```python
from build123d import *

# Parameters (mm, degrees)
SKETCH021_W             = 85.5
SKETCH021_H             = 85.5
SKETCH021_W_2           = 73.5
SKETCH021_H_2           = 73.5
PAD009006_DEPTH         = 11
SKETCH022_W             = 85.5
SKETCH022_H             = 85.5
SKETCH022_R             = 25.5
PAD009007_DEPTH         = 2
SKETCH023_R             = 1.5
POCKET003002_DEPTH      = 13.001
SKETCH024_R             = 1.5
POCKET003003_DEPTH      = 5
FILLET003_R             = 3
SKETCH025_W             = 45.5
SKETCH025_H             = 5
POCKET003004_DEPTH      = 85.501
POCKET003004_DEPTH_BACK = 0.001
SKETCH026_W             = 45.5
SKETCH026_H             = 5
POCKET003005_DEPTH      = 85.501


with BuildPart() as part:
    # Sketch021 → Pad009006 (new body)
    with BuildSketch(Plane.XY):
        Rectangle(SKETCH021_W, SKETCH021_H)
        Rectangle(SKETCH021_W_2, SKETCH021_H_2, mode=Mode.SUBTRACT)
    extrude(amount=PAD009006_DEPTH)

    # Sketch022 (on Face10 of Pad009006) → Pad009007 (join)
    with BuildSketch(Plane.XY.offset(11)):
        Rectangle(SKETCH022_W, SKETCH022_H)
        Circle(SKETCH022_R, mode=Mode.SUBTRACT)
    extrude(amount=PAD009007_DEPTH)

    # Sketch023 (on Face4 of Pad009007) → Pocket003002 (cut, through all)
    with BuildSketch(Plane(origin=(0, 0, 0), x_dir=(1, 0, 0), z_dir=(0, 0, -1))):
        with Locations((-39.235281, 39.235281)):
            Circle(SKETCH023_R)
        with Locations((39.235281, 39.235281)):
            Circle(SKETCH023_R)
        with Locations((39.235281, -39.235281)):
            Circle(SKETCH023_R)
        with Locations((-39.235281, -39.235281)):
            Circle(SKETCH023_R)
    extrude(amount=-POCKET003002_DEPTH, mode=Mode.SUBTRACT)

    # Sketch024 (on Face17 of Pocket003002) → Pocket003003 (cut)
    with BuildSketch(Plane.XY.offset(13)):
        with Locations((-30, 30)):
            Circle(SKETCH024_R)
        with Locations((30, 30)):
            Circle(SKETCH024_R)
        with Locations((30, -30)):
            Circle(SKETCH024_R)
        with Locations((-30, -30)):
            Circle(SKETCH024_R)
    extrude(amount=-POCKET003003_DEPTH, mode=Mode.SUBTRACT)

    # Fillet003
    fillet003_edges = [part.edges().sort_by_distance(p)[0] for p in [
        (42.75, 42.75, 5.5),
        (-42.75, 42.75, 5.5),
        (-42.75, -42.75, 5.5),
        (42.75, -42.75, 5.5),
    ]]
    fillet(fillet003_edges, radius=FILLET003_R)

    # Sketch025 (on Face1 of Fillet003) → Pocket003004 (cut, two sides)
    with BuildSketch(Plane(origin=(0, 42.75, 0), x_dir=(-1, 0, 0), z_dir=(0, 1, 0))) as pocket003004_sk:
        with Locations((0, 2.5)):
            Rectangle(SKETCH025_W, SKETCH025_H)
    extrude(amount=-POCKET003004_DEPTH, mode=Mode.SUBTRACT)
    extrude(pocket003004_sk.sketch, amount=POCKET003004_DEPTH_BACK, mode=Mode.SUBTRACT)

    # Sketch026 (on Face19 of Pocket003004) → Pocket003005 (cut, through all)
    with BuildSketch(Plane.YZ.offset(42.75)):
        with Locations((0, 2.5)):
            Rectangle(SKETCH026_W, SKETCH026_H)
    extrude(amount=-POCKET003005_DEPTH, mode=Mode.SUBTRACT)


solid = part.part
```
Geometry check sheet. Reference: the model listing, model coordinates, mm. A direction names the side the tool comes from. Give positions to 0.01 mm unless a question says otherwise; leave off trailing zeros. Write each loop counter-clockwise with the first axis right and the second up, starting at its lowest first coordinate (ties: lowest second). Pieces come first, ordered by that corner, then holes.
1) Section check A-A, the plane y = -30. Record the boundary of the cut face in (x, z).
2) Access from +Z, -Z, +X, -X, +Y, -Y to the whole of each face (thin tool, end or side, straight path). Record for faces 5 (the flat face through (0, 40, 5)), 6 (the flat face through (-36.75, -1, 7)), 7 (the flat face through (40, 22.75, 2)).
3) Gauge pin test, flat ends, axial feed: pin 1 (3.5 mm diameter, centred on x = 30, y = 30, fed in from -Z); pin 2 (5 mm diameter, centred on x = -38.5, y = -10, fed in from -Z); pin 3 (1.8 mm diameter, centred on x = -39.24, y = -39.24, fed in from +Z); pin 4 (1.5 mm diameter, centred on y = -41, z = 2, fed in from +X). Record the tip position at first contact, or that the pin passes through.
4) Material ranges on L1, parallel to Y at x = -30, z = 12; L2, parallel to Y at x = 0, z = 12.6; L3, parallel to X at y = -27.5, z = 8.5, recorded low to high.
5) Section check C-C, the plane y = 0. Record the boundary of the cut face in (x, z), and give its area (3 significant figures).
6) Release check for a two-part mould opening along Y. For faces 1 (the cylindrical face through (-41.89, -41.85, 6.59)), 2 (the flat face through (-1, -36.75, 7)), 3 (the flat face through (-22.75, 40, 2)), 4 (the flat face through (-1, 42.75, 8)) record: pulls with the +Y half, pulls with the -Y half, needs draft (parallel to the pull), parting line crosses it, or undercut.
Computed:
1. outline: (-42.75, 0) - (-36.75, 0) - (-36.75, 11) - (-31.5, 11) - (-31.5, 13) - (-42.75, 13) - close; (-28.5, 11) - (28.5, 11) - (28.5, 13) - (-28.5, 13) - close; (31.5, 11) - (36.75, 11) - (36.75, 0) - (42.75, 0) - (42.75, 13) - (31.5, 13) - close
2. face 5: -Z, +Y, -Y
2. face 6: -Z
2. face 7: -Z, +X, -X
3. pin 1: stops at z = 11
3. pin 2: stops at z = 5
3. pin 3: passes through
3. pin 4: stops at x = 42.71
4. L1: y = -42.75 to -31.5, -28.5 to 28.5, 31.5 to 42.75
4. L2: y = -42.75 to -25.5, 25.5 to 42.75
4. L3: x = -42.75 to -36.75, 36.75 to 42.75
5. outline: (-42.75, 5) - (-36.75, 5) - (-36.75, 11) - (-25.5, 11) - (-25.5, 13) - (-42.75, 13) - close; (25.5, 11) - (36.75, 11) - (36.75, 5) - (42.75, 5) - (42.75, 13) - (25.5, 13) - close
5. area: 141 mm2
6. face 1: pulls with the -Y half
6. face 2: undercut
6. face 3: needs draft
6. face 4: pulls with the +Y half
